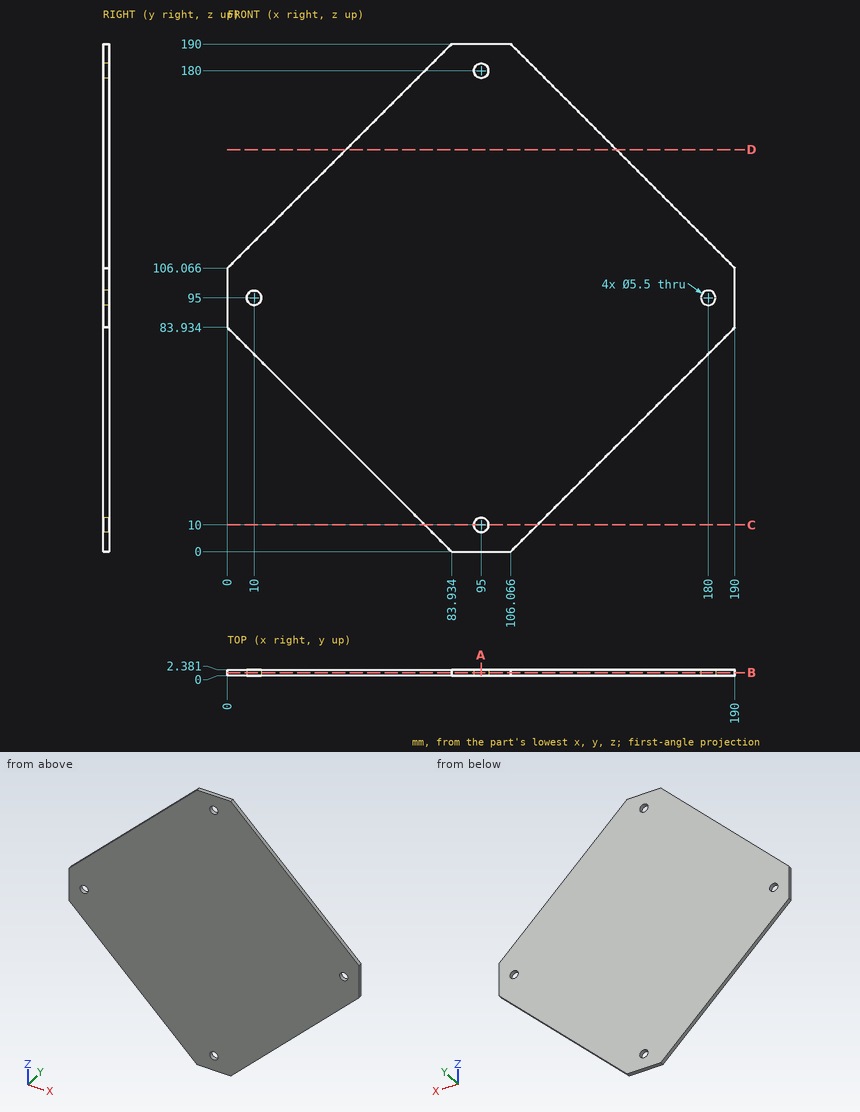
Input: dimensioned drawing with shaded views. Units: mm. Origin: part minimum x, y, z. Give positions to 0.01 mm unless a question says otherwise; leave off trailing zeros. Loops run counter-clockwise (first coordinate to the right, second up) from the corner with the lowest first, then second, coordinate; pieces in that order, holes last. Notation, with made-up numbers: M -2,89.25 L 52,89.25 A32 ccw 52,120.25 Z; hole C -34,56.5 d7. An arc over 180 degrees is marked long. Put each result on its own line as item: value.
1) Material intervals for L1, parallel to X at y = 1.25, z = 19 (1 decimal); L2, parallel to Z at x = 74.5, y = 2.25 (1 decimal); L3, parallel to X at y = 1.7, z = 157 (1 decimal), sorted ascending. Write a range as from..to.
Computed values:
L1: x = 64.9..125.1
L2: z = 9.4..180.6
L3: x = 50.9..139.1
2) Cut plane D-D, the plane z = 150.5. Return the cut outline in (x, y), plus the area to 3 significant figures.
Computed values:
outline: M 44.43,0 L 145.57,0 L 145.57,2.38 L 44.43,2.38 Z
area: 241 mm^2
3) Cut plane C-C, the plane z = 10. Return the cut outline in (x, y).
Computed values:
outline: M 73.93,0 L 92.25,0 L 92.25,2.38 L 73.93,2.38 Z; M 97.75,0 L 116.07,0 L 116.07,2.38 L 97.75,2.38 Z
4) Cut plane A-A, the plane x = 95. Return the cut outline in (y, z), plus the area to 3 significant figures.
Computed values:
outline: M 0,0 L 2.38,0 L 2.38,7.25 L 0,7.25 Z; M 0,12.75 L 2.38,12.75 L 2.38,177.25 L 0,177.25 Z; M 0,182.75 L 2.38,182.75 L 2.38,190 L 0,190 Z
area: 426 mm^2
5) Cut plane B-B, the plane y = 1.25. Return the cut outline in (x, z), plus the area to 3 significant figures.
Computed values:
outline: M 0,83.93 L 83.93,0 L 106.07,0 L 190,83.93 L 190,106.07 L 106.07,190 L 83.93,190 L 0,106.07 Z; hole C 10,95 d5.5; hole C 95,10 d5.5; hole C 95,180 d5.5; hole C 180,95 d5.5
area: 21,900 mm^2
